Source: CAD feature listing. Evaluate the final solid. Frame: model axes, mm. A direction names the side the tool comes from. Give positions to 0.01 mm unless a question says otherwise; leave off trailing zeros. Loops run counter-clockwise (first coordinate to the right, second up) from the corner with the lowest first, then second, coordinate; pieces in that order, holes last. Notation, with made-up numbers: M -15,28.25 L 26,28.25 A14 ccw 26,47.25 Z; hole C 66,39 d11. An arc over 180 degrees is marked long. Put each result on its own line as item: value.
from build123d import *

# Parameters (mm, degrees)
SKETCH_1_W          = 40
SKETCH_1_H          = 80
EXTRUDE_1_DEPTH     = 20
SKETCH_2_W          = 40
SKETCH_2_H          = 25
EXTRUDE_2_DEPTH     = 20
SKETCH_3_R          = 3.87339884
SKETCH_3_R_2        = 6.424173687
CUT_EXTRUDE_1_DEPTH = 5


with BuildPart() as part:
    # 草图1 → 凸台-拉伸1 (new body)
    with BuildSketch(Plane.XY):
        Rectangle(SKETCH_1_W, SKETCH_1_H)
    extrude(amount=EXTRUDE_1_DEPTH)

    # 草图2 → 凸台-拉伸2 (add)
    with BuildSketch(Plane.XY.offset(20)):
        with Locations((0, 27.5)):
            Rectangle(SKETCH_2_W, SKETCH_2_H)
    extrude(amount=EXTRUDE_2_DEPTH)

    # 草图3 → 切除-拉伸1 (cut)
    with BuildSketch(Plane(origin=(0, 40, 0), x_dir=(1, 0, 0), z_dir=(0, 1, 0))):
        with Locations(Location((-10.297572527, -17.722901183, 0), (0, 0, 270))):
            Circle(SKETCH_3_R)
        with Locations(Location((6.329700544, -18.573159465, 0), (0, 0, 270))):
            Circle(SKETCH_3_R_2)
    extrude(amount=-CUT_EXTRUDE_1_DEPTH, mode=Mode.SUBTRACT)


solid = part.part
1. Section query B-B (y = -22.5). Output: boundary loops of the cut face in (x, z).
Found:
outline: M -20,0 L 20,0 L 20,20 L -20,20 Z
2. Draft query along Z for faces 4 (the flat face through (0, 28, 40)), 5 (the flat face through (-0.3, 40, 19.7)), 6 (the flat face through (-10, 35, 18)). Return one class per face: pulls with the +Z half, pulls with the -Z half, needs draft (parallel to the pull), parting line crosses it, or undercut.
Found:
face 4: pulls with the +Z half
face 5: needs draft
face 6: undercut
3. Section query D-D (x = 8.5). Output: boundary loops of the cut face in (y, z), plus the area to 3 significant figures.
Found:
outline: M -40,0 L 40,0 L 40,12.53 L 35,12.53 L 35,24.62 L 40,24.62 L 40,40 L 15,40 L 15,20 L -40,20 Z
area: 2,040 mm^2
4. Contact query for flat-ended pins moving along their axis: P1, Ø1, axis at x = -15.5, z = 33.5, coming from the -Y side; P2, Ø6, axis at x = -10.3, z = 17.72, coming from the +Y side; P3, Ø6, axis at x = 9, y = -1, coming from the +Z side. Output: stop coordinate, or through.
Found:
P1: y = 15
P2: y = 35
P3: z = 20
5. Section query C-C (z = 32.5). Output: boundary loops of the cut face in (x, y), plus the area to 3 significant figures.
Found:
outline: M -20,15 L 20,15 L 20,40 L -20,40 Z
area: 1,000 mm^2
6. Access query for faces 1 (the flat face through (0, -12, 20)), 2 (the flat face through (0, -40, 10)), 3 (the flat face through (6, 35, 18)). Directions: +Z, -Z, +X, -X, +Y, -Y. A direction counts if a zero-diameter tool reaches every point of the face in a straight line with its end or side. Return the directions, or none.
Found:
face 1: +Z, +X, -X, -Y
face 2: +Z, -Z, +X, -X, -Y
face 3: +Y
7. Section query A-A (x = -4). Output: boundary loops of the cut face in (y, z), plus the area to 3 significant figures.
Found:
outline: M -40,0 L 40,0 L 40,40 L 15,40 L 15,20 L -40,20 Z
area: 2,100 mm^2
8. Material intervals for line 1 (Y direction, x = -11, z = 16.5); line 2 (Z direction, x = 16.5, y = -26.5); line 3 (Y direction, x = 3.5, z = 22.5), sorted ascending. Write a range as from..to.
Found:
line 1: -40..35
line 2: 0..20
line 3: 15..35
